Check sheet for the modelled part. Datum: model origin and axes. Units: mm. Round coordinates to 2 decimals unless told otherwise and drop trailing zeros. Write each loop counter-clockwise with the first axis right and the second up, starting at its lowest first coordinate (ties: lowest second). Pieces come first, ordered by that corner, then holes. Notation, with made-up numbers: (76, 38) -> (98, 38) arc R12 cw to (98, 47) -> close; hole circle Ø2 at (24.5, -9.75). An arc over 180 degrees is marked (long way). Write item = value, one per line.
from build123d import *

# Parameters (mm, degrees)
F1_DEPTH = 101.6
F0_W     = 25.4
F0_H     = 25.4
F0_R     = 3.81
F2_DEPTH = 3.175


# Not quite as in the source:
# - a feature names something its author has since deleted; it is built from what else it names


with BuildPart() as f1:
    # F0 (on Front) → F1 (new body)
    with BuildSketch(Plane.XZ):
        Polygon((0, 25.4), (0, 0), (3.175, 0), (3.175, 1828.8), (1222.375, 1828.8), (1222.375, 0), (1225.55, 0), (1225.55, 25.4), (1225.55, 50.8), (1225.55, 318.0291666667), (1225.55, 343.4291666667), (1225.55, 610.6583333333), (1225.55, 636.0583333333), (1225.55, 903.2875), (1225.55, 928.6875), (1225.55, 1195.9166666667), (1225.55, 1221.3166666667), (1225.55, 1488.5458333333), (1225.55, 1513.9458333333), (1225.55, 1781.175), (1225.55, 1806.575), (1225.55, 1831.975), (1200.15, 1831.975), (1174.75, 1831.975), (912.8125, 1831.975), (887.4125, 1831.975), (625.475, 1831.975), (600.075, 1831.975), (338.1375, 1831.975), (312.7375, 1831.975), (50.8, 1831.975), (25.4, 1831.975), (0, 1831.975), (0, 1806.575), (0, 1781.175), (0, 1513.9458333333), (0, 1488.5458333333), (0, 1221.3166666667), (0, 1195.9166666667), (0, 928.6875), (0, 903.2875), (0, 636.0583333333), (0, 610.6583333333), (0, 343.4291666667), (0, 318.0291666667), (0, 50.8), align=None)
    extrude(amount=F1_DEPTH)

    # F0 (on Front) → F2 (join)
    with BuildSketch(Plane.XZ):
        with Locations((-12.7, 38.1)):
            Rectangle(F0_W, F0_H)
        with Locations((-12.7, 38.1)):
            Circle(F0_R, mode=Mode.SUBTRACT)
        with Locations((-12.7, 330.7291666667)):
            Rectangle(F0_W, F0_H)
        with Locations((-12.7, 330.7291666667)):
            Circle(F0_R, mode=Mode.SUBTRACT)
        with Locations((-12.7, 623.3583333333)):
            Rectangle(F0_W, F0_H)
        with Locations((-12.7, 623.3583333333)):
            Circle(F0_R, mode=Mode.SUBTRACT)
        with Locations((1238.25, 38.1)):
            Rectangle(F0_W, F0_H)
        with Locations((1238.25, 38.1)):
            Circle(F0_R, mode=Mode.SUBTRACT)
        with Locations((-12.7, 915.9875)):
            Rectangle(F0_W, F0_H)
        with Locations((-12.7, 915.9875)):
            Circle(F0_R, mode=Mode.SUBTRACT)
        with Locations((1238.25, 330.7291666667)):
            Rectangle(F0_W, F0_H)
        with Locations((1238.25, 330.7291666667)):
            Circle(F0_R, mode=Mode.SUBTRACT)
        with Locations((-12.7, 1208.6166666667)):
            Rectangle(F0_W, F0_H)
        with Locations((-12.7, 1208.6166666667)):
            Circle(F0_R, mode=Mode.SUBTRACT)
        with Locations((1238.25, 623.3583333333)):
            Rectangle(F0_W, F0_H)
        with Locations((1238.25, 623.3583333333)):
            Circle(F0_R, mode=Mode.SUBTRACT)
        with Locations((-12.7, 1501.2458333333)):
            Rectangle(F0_W, F0_H)
        with Locations((-12.7, 1501.2458333333)):
            Circle(F0_R, mode=Mode.SUBTRACT)
        with Locations((1238.25, 915.9875)):
            Rectangle(F0_W, F0_H)
        with Locations((1238.25, 915.9875)):
            Circle(F0_R, mode=Mode.SUBTRACT)
        with Locations((-12.7, 1793.875)):
            Rectangle(F0_W, F0_H)
        with Locations((-12.7, 1793.875)):
            Circle(F0_R, mode=Mode.SUBTRACT)
        with Locations((1238.25, 1208.6166666667)):
            Rectangle(F0_W, F0_H)
        with Locations((1238.25, 1208.6166666667)):
            Circle(F0_R, mode=Mode.SUBTRACT)
        with Locations((38.1, 1844.675)):
            Rectangle(F0_W, F0_H)
        with Locations((38.1, 1844.675)):
            Circle(F0_R, mode=Mode.SUBTRACT)
        with Locations((1238.25, 1501.2458333333)):
            Rectangle(F0_W, F0_H)
        with Locations((1238.25, 1501.2458333333)):
            Circle(F0_R, mode=Mode.SUBTRACT)
        with Locations((325.4375, 1844.675)):
            Rectangle(F0_W, F0_H)
        with Locations((325.4375, 1844.675)):
            Circle(F0_R, mode=Mode.SUBTRACT)
        with Locations((1238.25, 1793.875)):
            Rectangle(F0_W, F0_H)
        with Locations((1238.25, 1793.875)):
            Circle(F0_R, mode=Mode.SUBTRACT)
        with Locations((612.775, 1844.675)):
            Rectangle(F0_W, F0_H)
        with Locations((612.775, 1844.675)):
            Circle(F0_R, mode=Mode.SUBTRACT)
        with Locations((1187.45, 1844.675)):
            Rectangle(F0_W, F0_H)
        with Locations((1187.45, 1844.675)):
            Circle(F0_R, mode=Mode.SUBTRACT)
        with Locations((900.1125, 1844.675)):
            Rectangle(F0_W, F0_H)
        with Locations((900.1125, 1844.675)):
            Circle(F0_R, mode=Mode.SUBTRACT)
    extrude(amount=F2_DEPTH)


solid = f1.part
(1) Material ranges on L1, parallel to X at y = -76, z = 1078.5 (3 decimals); L2, parallel to Z at x = 272, y = -83 (3 decimals), recorded low to high. Write a range as [from, to].
Worked answers:
L1 = [0, 3.175], [1222.375, 1225.55]
L2 = [1828.8, 1831.975]
(2) Sectioned sample at C-C on x = 92. Enter the section's corners in (y, z) (3 decimals), then the cut area to 3 significant figures.
Worked answers:
outline = (-101.6, 1828.8) -> (0, 1828.8) -> (0, 1831.975) -> (-101.6, 1831.975) -> close
area = 323 mm²
(3) Go/stop test with flat-tipped pins: P1, Ø2.5, axis at y = -1, z = 1845.5, coming from the -X side; P2, Ø2, axis at x = 610.5, y = -19, coming from the +Z side (3 decimals); P3, Ø7, axis at x = 1187.45, z = 1844.675, coming from the -Y side; P4, Ø3.5, axis at x = 1243, y = -1.5, coming from the -Z side. Record where each tip stops, or that it passes through.
Worked answers:
P1 = 25.4
P2 = 1831.975
P3 = through
P4 = 25.4
(4) Sectioned sample at A-A on z = 1448. Enter the section's corners in (x, y) (3 decimals).
Worked answers:
outline = (0, -101.6) -> (3.175, -101.6) -> (3.175, 0) -> (0, 0) -> close; (1222.375, -101.6) -> (1225.55, -101.6) -> (1225.55, 0) -> (1222.375, 0) -> close
(5) Release check for a two-part mould opening along X. For faces 1 (the flat face through (3.175, -50, 902)), 2 (the flat face through (1225.55, -50, 903)), 3 (the flat face through (1224, 0, 933)) record: pulls with the +X half, pulls with the -X half, needs draft (parallel to the pull), parting line crosses it, or undercut.
Worked answers:
face_1 = undercut
face_2 = pulls with the +X half
face_3 = needs draft
(6) Sectioned sample at B-B on y = -51.5. Enter the section's corners in (x, z) (3 decimals).
Worked answers:
outline = (0, 0) -> (3.175, 0) -> (3.175, 1828.8) -> (1222.375, 1828.8) -> (1222.375, 0) -> (1225.55, 0) -> (1225.55, 1831.975) -> (0, 1831.975) -> close
